The listing builds one solid part. Answer for the finished solid, in the listing's coordinates (mm). Face numbers are marked on the shaded views. A direction names the side the tool comes from. Give positions to 0.01 mm unless a question says otherwise; leave off trailing zeros. Write each loop counter-clockwise with the first axis right and the second up, starting at its lowest first coordinate (ties: lowest second). Pieces come first, ordered by that corner, then holes.
```python
from build123d import *

# Parameters (mm, degrees)
F0_W      = 19.06034071
F0_H      = 19.06034071
F1_DEPTH  = 9.525
F2_R      = 1.8892312699
F8_DEPTH  = 0.254
F3_R      = 1.7327827713
F9_DEPTH  = 0.254
F4_R      = 2.1821211745
F10_DEPTH = 0.254
F5_R      = 2.0368058648
F11_DEPTH = 0.254
F6_R      = 1.8590976902
F12_DEPTH = 0.254
F7_R      = 2.1308019233
F7_R_2    = 2.1821211745
F13_DEPTH = 0.254


with BuildPart() as f1:
    # F0 (on Front) → F1 (new body, symmetric)
    with BuildSketch(Plane.XZ):
        with Locations((11.5190818906, 14.3221947365)):
            Rectangle(F0_W, F0_H)
    extrude(amount=F1_DEPTH, both=True)

    # F2 (on face) → F8 (join)
    with BuildSketch(Plane(origin=(1.9889115356, 0, 0), x_dir=(0, -1, 0), z_dir=(-1, 0, 0))):
        with Locations((0, 14.4774196669)):
            Circle(F2_R)
    extrude(amount=F8_DEPTH)

    # F3 (on face) → F9 (join)
    with BuildSketch(Plane.YZ.offset(21.0492522456)):
        with Locations((-4.953, 19.2803650914)):
            Circle(F3_R)
        with Locations((4.953, 19.2803650914)):
            Circle(F3_R)
        with Locations((4.953, 10.1363650914)):
            Circle(F3_R)
        with Locations((-4.953, 10.1363650914)):
            Circle(F3_R)
        with Locations((-4.953, 14.7083650914)):
            Circle(F3_R)
        with Locations((4.953, 14.7083650914)):
            Circle(F3_R)
    extrude(amount=F9_DEPTH)

    # F4 (on face) → F10 (join)
    with BuildSketch(Plane(origin=(0, 9.525, 0), x_dir=(-1, 0, 0), z_dir=(0, 1, 0))):
        with Locations((-16.2232522456, 19.0263650914)):
            Circle(F4_R)
        with Locations((-6.8149115356, 9.6180243815)):
            Circle(F4_R)
    extrude(amount=F10_DEPTH)

    # F5 (on face) → F11 (join)
    with BuildSketch(Plane.XY.offset(23.8523650914)):
        with Locations((16.7312522456, -5.207)):
            Circle(F5_R)
        with Locations((11.5242522456, 0)):
            Circle(F5_R)
        with Locations((6.3069115356, 5.207)):
            Circle(F5_R)
    extrude(amount=F11_DEPTH)

    # F6 (on face) → F12 (join)
    with BuildSketch(Plane(origin=(0, 0, 4.7920243815), x_dir=(1, 0, 0), z_dir=(0, 0, -1))):
        with Locations((5.7989115356, 5.715)):
            Circle(F6_R)
        with Locations((17.2392522456, 5.715)):
            Circle(F6_R)
        with Locations((5.7989115356, -5.715)):
            Circle(F6_R)
        with Locations((17.2392522456, -5.715)):
            Circle(F6_R)
    extrude(amount=F12_DEPTH)

    # F7 (on face) → F13 (join)
    with BuildSketch(Plane.XZ.offset(9.525)):
        with Locations((5.7989115356, 8.6020243815)):
            Circle(F7_R)
        with Locations((17.2392522456, 20.0423650914)):
            Circle(F7_R_2)
        with Locations((5.7989115356, 20.0423650914)):
            Circle(F7_R_2)
        with Locations((17.2392522456, 8.6020243815)):
            Circle(F7_R_2)
        with Locations((11.5139115356, 14.3170229782)):
            Circle(F7_R_2)
    extrude(amount=F13_DEPTH)


solid = f1.part
```
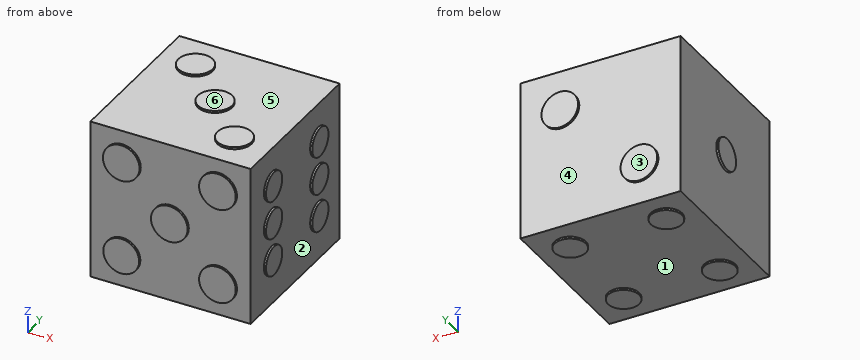
Item 1: A cutting plane is placed at B-B, the plane x = 5. Give the vertices of the cut face in (y, z) (3 decimals), plus the area to 3 significant figures.
Conclusion:
outline: (-9.779, 6.627) - (-9.525, 6.627) - (-9.525, 4.792) - (-7.394, 4.792) - (-7.394, 4.538) - (-4.036, 4.538) - (-4.036, 4.792) - (4.036, 4.792) - (4.036, 4.538) - (7.394, 4.538) - (7.394, 4.792) - (9.525, 4.792) - (9.525, 8.407) - (9.779, 8.407) - (9.779, 10.83) - (9.525, 10.83) - (9.525, 23.852) - (6.769, 23.852) - (6.769, 24.106) - (3.645, 24.106) - (3.645, 23.852) - (-9.525, 23.852) - (-9.525, 22.073) - (-9.779, 22.073) - (-9.779, 18.012) - (-9.525, 18.012) - (-9.525, 10.577) - (-9.779, 10.577) - close
area: 368 mm2
Item 2: Which of the six approach directions +Z, -Z, +X, -X, +Y, -Y give full straight-line access (tool end or side, diameter ignored) to the marked faces 4, 5 and 6?
Conclusion:
face 4: +Y
face 5: +Z
face 6: +Z, +X, -X, +Y, -Y
Item 3: Each of these flat-tipped pins is pushed along its axis until it touches: P1, Ø5.5, axis at y = 0, z = 18.5, coming from the -X side; P2, Ø3, axis at x = 15, y = 2, coming from the -Z side; P3, Ø4, axis at x = 18.5, z = 11.5, coming from the +Y side (3 decimals); P4, Ø1.5, axis at y = -0.5, z = 10, coming from the +X side. Where does it stop, or does it pass through?
Conclusion:
P1: stops at x = 1.73
P2: stops at z = 4.79
P3: stops at y = 9.525
P4: stops at x = 21.05
Item 4: Consider probe 1 along Z at (x, y) = (4.75, 3); probe 2 along Y at (x, z) = (14, 9.75) (3 decimals); probe 3 along Y at (x, z) = (12.5, 12.5) (3 decimals). Determine where each line is inside the solid, lowest interval first.
Conclusion:
probe 1: z = 4.79 to 23.85
probe 2: y = -9.525 to 9.525
probe 3: y = -9.779 to 9.525
Item 5: A cutting plane is placed at C-C, the plane z = 18.25. Give the vertices of the cut face in (x, y) (3 decimals).
Conclusion:
outline: (1.989, -9.525) - (4.554, -9.525) - (4.554, -9.779) - (7.044, -9.779) - (7.044, -9.525) - (15.995, -9.525) - (15.995, -9.779) - (18.484, -9.779) - (18.484, -9.525) - (21.049, -9.525) - (21.049, -6.346) - (21.303, -6.346) - (21.303, -3.56) - (21.049, -3.56) - (21.049, 3.56) - (21.303, 3.56) - (21.303, 6.346) - (21.049, 6.346) - (21.049, 9.525) - (18.263, 9.525) - (18.263, 9.779) - (14.184, 9.779) - (14.184, 9.525) - (1.989, 9.525) - close
Item 6: Determine the mould class of the marked faces 1, 2 and 3 for opening direction X: pulls with the +X half, pulls with the -X half, needs draft (parallel to the pull), parting line crosses it, or undercut.
Conclusion:
face 1: undercut
face 2: pulls with the +X half
face 3: needs draft
Item 7: A cutting plane is placed at D-D, the plane y = 4.5. Give the vertices of the cut face in (x, z), plus the area to 3 significant figures.
Conclusion:
outline: (1.99, 4.79) - (4.39, 4.79) - (4.39, 4.54) - (7.21, 4.54) - (7.21, 4.79) - (15.83, 4.79) - (15.83, 4.54) - (18.65, 4.54) - (18.65, 4.79) - (21.05, 4.79) - (21.05, 8.46) - (21.3, 8.46) - (21.3, 11.81) - (21.05, 11.81) - (21.05, 13.04) - (21.3, 13.04) - (21.3, 16.38) - (21.05, 16.38) - (21.05, 17.61) - (21.3, 17.61) - (21.3, 20.95) - (21.05, 20.95) - (21.05, 23.85) - (8.22, 23.85) - (8.22, 24.11) - (4.4, 24.11) - (4.4, 23.85) - (1.99, 23.85) - close
area: 368 mm2
Item 8: A cutting plane is placed at A-A, the plane y = 0. Give the vertices of the cut face in (x, z).
Conclusion:
outline: (1.73, 12.59) - (1.99, 12.59) - (1.99, 4.79) - (21.05, 4.79) - (21.05, 23.85) - (13.56, 23.85) - (13.56, 24.11) - (9.49, 24.11) - (9.49, 23.85) - (1.99, 23.85) - (1.99, 16.37) - (1.73, 16.37) - close
